```python
from build123d import *

# Parameters (mm, degrees)
F0_W     = 404
F0_H     = 145
F0_R     = 2.5
F0_R_2   = 1.5
F0_W_2   = 53.5
F0_H_2   = 13
F0_R_3   = 3.25
F0_W_3   = 7
F0_H_3   = 14.5
F0_R_4   = 8
F0_R_5   = 1.75
F1_DEPTH = 2


with BuildPart() as f1:
    # F0 (on Top) → F1 (new body)
    with BuildSketch(Plane.XY):
        Rectangle(F0_W, F0_H)
        with Locations((-196.113765, -60.5)):
            Circle(F0_R, mode=Mode.SUBTRACT)
        with Locations((-187, -57.5)):
            Circle(F0_R_2, mode=Mode.SUBTRACT)
        with Locations((-159.75, -44)):
            Rectangle(F0_W_2, F0_H_2, mode=Mode.SUBTRACT)
        with Locations((-73, -57.5)):
            Circle(F0_R_2, mode=Mode.SUBTRACT)
        with Locations((-100.25, -44)):
            Rectangle(F0_W_2, F0_H_2, mode=Mode.SUBTRACT)
        with Locations((-42.060282, -46.764122)):
            Circle(F0_R_3, mode=Mode.SUBTRACT)
        with Locations((-42.060282, -21.764122)):
            Circle(F0_R_3, mode=Mode.SUBTRACT)
        with Locations((-42.060282, 3.235878)):
            Circle(F0_R_3, mode=Mode.SUBTRACT)
        with Locations((-42.060282, 28.235878)):
            Circle(F0_R_3, mode=Mode.SUBTRACT)
        with Locations((-186.5, 37.4)):
            Circle(F0_R_2, mode=Mode.SUBTRACT)
        with Locations((-186.5, 52.45)):
            Rectangle(F0_W_3, F0_H_3, mode=Mode.SUBTRACT)
        with Locations((-186.5, 67.5)):
            Circle(F0_R_2, mode=Mode.SUBTRACT)
        with Locations((-42.060282, 53.235878)):
            Circle(F0_R_3, mode=Mode.SUBTRACT)
        with Locations((0, 28.235878)):
            Circle(F0_R_3, mode=Mode.SUBTRACT)
        with Locations((0, 53.235878)):
            Circle(F0_R_4, mode=Mode.SUBTRACT)
        with Locations((148, 57.5)):
            Circle(F0_R_5, mode=Mode.SUBTRACT)
        with BuildLine():
            ThreePointArc((182, 51.5), (180.828427, 48.671573), (178, 47.5))
            Line((178, 47.5), (158, 47.5))
            ThreePointArc((158, 47.5), (155.171573, 48.671573), (154, 51.5))
            Line((154, 51.5), (154, 63.5))
            ThreePointArc((154, 63.5), (155.171573, 66.328427), (158, 67.5))
            Line((158, 67.5), (178, 67.5))
            ThreePointArc((178, 67.5), (180.828427, 66.328427), (182, 63.5))
            Line((182, 63.5), (182, 51.5))
        make_face(mode=Mode.SUBTRACT)
        with Locations((188, 57.5)):
            Circle(F0_R_5, mode=Mode.SUBTRACT)
    extrude(amount=-F1_DEPTH)


solid = f1.part
```
The listing builds one solid part. Answer for the finished solid, in the listing's coordinates (mm). Give positions to 0.01 mm unless a question says otherwise; leave off trailing zeros. Order: outer loops, then holes, each group sorted by start corner. A loop starts at its lowest first (then second) coordinate and runs counter-clockwise, first axis right, second up. Notation, with made-up numbers: (-16, 8.25) -> (38, 8.25) arc R9 cw to (38, 14.25) -> close; hole circle Ø5 at (8, 35). An arc over 180 degrees is marked (long way). Answer as a JSON object with one key per item and string values. Group by question number.
Item 1: The part is cut by section B-B on z = -1.6. Give the number of separate pieces and of enclosed holes in the cut face, and give its area (3 significant figures).
Item 2: Consider L1, parallel to Y at x = 0, z = -0.7; L2, parallel to Y at x = 148, z = -1.2; L3, parallel to Y at x = -88.5, z = -1.7. Determine where each line is inside the solid, lowest interval first. Write a range as from..to.
Item 3: The part is cut by section A-A on x = -95.5. Write down the section's boundary in (y, z).
Item 4: A flat-ended cylindrical pin translates along its axis: pin 1 (4 mm diameter, centred on x = -42.06, y = 28.24, fed in from -Z). Find the tip coordinate at first contact, or state that the pin passes through.
Item 5: Determine the mould class of faces 1 (the cylindrical face through (-1.734, 45.426, -0.986)), 2 (the cylindrical face through (-42.765, 25.063, -0.986)), 3 (the flat face through (-3, 1, -2)) for opening direction Y: pulls with the +Y half, pulls with the -Y half, needs draft (parallel to the pull), parting line crosses it, or undercut.
Result set:
{
 "1": {"separate pieces": "1", "enclosed holes": "18", "area": "56,100 mm²"},
 "2": {"L1": "-72.5..24.99, 31.49..45.24, 61.24..72.5", "L2": "-72.5..55.75, 59.25..72.5", "L3": "-72.5..-50.5, -37.5..72.5"},
 "3": {"outline": "(-72.5, -2) -> (-50.5, -2) -> (-50.5, 0) -> (-72.5, 0) -> close; (-37.5, -2) -> (72.5, -2) -> (72.5, 0) -> (-37.5, 0) -> close"},
 "4": {"pin 1": "through"},
 "5": {"face 1": "undercut", "face 2": "undercut", "face 3": "needs draft"}
}
